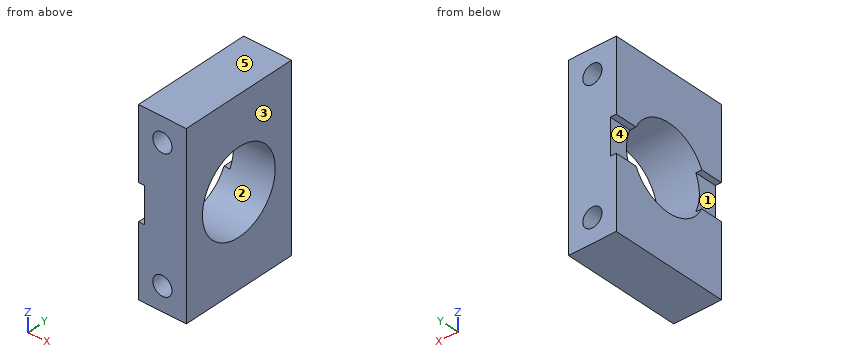
from build123d import *

# Parameters (mm, degrees)
SKETCH1_W           = 47.625
SKETCH1_H           = 31.75
SKETCH1_R           = 11
BOSS_EXTRUDE1_DEPTH = 6.35
SKETCH3_R           = 2.5527
CUT_EXTRUDE2_DEPTH  = 41.192289761
SKETCH4_W           = 9.525
SKETCH4_H           = 35.649275258
CUT_EXTRUDE3_DEPTH  = 1.5875


with BuildPart() as part:
    # Sketch1 → Boss-Extrude1 (new, symmetric)
    with BuildSketch(Plane(origin=(0, 0, 0), x_dir=(0, 0, -1), z_dir=(1, 0, 0))):
        Rectangle(SKETCH1_W, SKETCH1_H)
        Circle(SKETCH1_R, mode=Mode.SUBTRACT)
    extrude(amount=BOSS_EXTRUDE1_DEPTH, both=True)

    # Sketch3 → Cut-Extrude2 (cut, through all)
    with BuildSketch(Plane.XZ.offset(15.875)):
        with Locations(Location((0, 17.4625, 0), (0, 0, 270))):
            Circle(SKETCH3_R)
    cut_extrude2 = extrude(amount=-CUT_EXTRUDE2_DEPTH, mode=Mode.SUBTRACT)

    # Mirror1: Cut-Extrude2 across plane
    add(cut_extrude2.mirror(Plane.XY), mode=Mode.SUBTRACT)

    # Sketch4 → Cut-Extrude3 (cut)
    with BuildSketch(Plane.ZY.offset(6.35)):
        Rectangle(SKETCH4_W, SKETCH4_H)
    extrude(amount=-CUT_EXTRUDE3_DEPTH, mode=Mode.SUBTRACT)


solid = part.part
Model file for the job. Use its own axes, mm. Face numbers are marked on the shaded views. A direction names the side the tool comes from. Coordinates: 2 decimals unless noted, no trailing zeros. Order: outer loops, then holes, each group sorted by start corner. A loop starts at its lowest first (then second) coordinate and runs counter-clockwise, first axis right, second up. Notation, with made-up numbers: (-13.75, 32.5) -> (17.25, 32.5) arc R15 cw to (17.25, 60.5) -> close; hole circle Ø7 at (-23, 53.25). An arc over 180 degrees is marked (long way). Return JSON: item names as keys, results as strings. Group by question number.
Item 1: Flat gauge pins, fed straight in: P1, Ø5, axis at y = -12, z = -1, coming from the -X side; P2, Ø10, axis at y = -8.5, z = -6, coming from the +X side. Where does each tip first touch, or does it go through?
Item 2: Saw through at B-B on y = 0. Write the cut outline in (x, z).
Item 3: Wall check: line 1 along Z through (x, y) = (1.75, 8); line 2 along Z through (x, y) = (2, 2.5); line 3 along Y through (x, z) = (2.5, 0) (3 decimals). Give the ranges that are in metal, low to high. Write a range as [from, to].
Item 4: Saw through at D-D on y = 13. Write the cut outline in (x, z), then the cut area to 3 significant figures.
Item 5: Pull direction Z, two halves, no side cores. Call the marked faces 3, 4 and 5: pulls with the +Z half, pulls with the -Z half, needs draft (parallel to the pull), parting line crosses it, or undercut.
Item 6: Saw through at A-A on x = 0. Write the cut outline in (y, z) (1 decimal), then the cut area to 3 significant figures.
Item 7: Tool access for the marked faces 1 and 2: list every direction of +Z, -Z, +X, -X, +Y, -Y with a clear straight run to the whole face (end or side of a thin tool).
Values found:
{
 "1": {"P1": "stops at x = -4.76", "P2": "stops at x = 6.35"},
 "2": {"outline": "(-6.35, -23.81) -> (6.35, -23.81) -> (6.35, -11) -> (-6.35, -11) -> close; (-6.35, 11) -> (6.35, 11) -> (6.35, 23.81) -> (-6.35, 23.81) -> close; hole circle Ø5.11 at (0, -17.46); hole circle Ø5.11 at (0, 17.46)"},
 "3": {"line 1": "z = [-23.81, -19.32], [-15.6, -7.55], [7.55, 15.6], [19.32, 23.81]", "line 2": "z = [-23.81, -19.05], [-15.88, -10.71], [10.71, 15.88], [19.05, 23.81]", "line 3": "y = [-15.875, -11], [11, 15.875]"},
 "4": {"outline": "(-6.35, -23.81) -> (6.35, -23.81) -> (6.35, 23.81) -> (-6.35, 23.81) -> (-6.35, 4.76) -> (-4.76, 4.76) -> (-4.76, -4.76) -> (-6.35, -4.76) -> close; hole circle Ø5.11 at (0, -17.46); hole circle Ø5.11 at (0, 17.46)", "area": "549 mm2"},
 "5": {"face 3": "needs draft", "face 4": "undercut", "face 5": "pulls with the +Z half"},
 "6": {"outline": "(-15.9, -23.8) -> (15.9, -23.8) -> (15.9, -20) -> (-15.9, -20) -> close; (-15.9, -14.9) -> (15.9, -14.9) -> (15.9, 14.9) -> (-15.9, 14.9) -> close; (-15.9, 20) -> (15.9, 20) -> (15.9, 23.8) -> (-15.9, 23.8) -> close; hole circle Ø22 at (0, 0)", "area": "808 mm2"},
 "7": {"face 1": "-X, +Y, -Y", "face 2": "+X, -X"}
}
